Check sheet for the modelled part. Datum: model origin and axes. Units: mm. A direction names the side the tool comes from. Round coordinates to 2 decimals unless told otherwise and drop trailing zeros. Order: outer loops, then holes, each group sorted by start corner. A loop starts at its lowest first (then second) coordinate and runs counter-clockwise, first axis right, second up.
(1) Sectioned sample at C-C, the plane y = 14.75. Enter the section's corners in (x, z).
(2) Sectioned sample at B-B, the plane z = 0. Enter the section's corners in (x, y), and give its area (3 significant figures).
(3) Mould release check, pull along X, two halves, no side actions. Record for faces 3 (the cylindrical face through (15.51, -3.24, -3.44)), 4 (the flat face through (0, 0, 0)), 5 (the flat face through (7, -5.016, -13)): released by +X, released by -X, zero draft, split by the parting line, or undercut.
(4) Depth check by flat-ended pin: pin 1 (4 mm diameter, centred on x = 1.5, z = -4, fed in from +Y); pin 2 (6 mm diameter, centred on y = -0.5, z = 6, fed in from +X); pin 3 (6 mm diameter, centred on x = -7, z = -8, fed in from +Y); pin 4 (3 mm diameter, centred on x = -4, y = 9, fed in from -Z). Enter the tip coordinate at first touch or a pass-through.
(5) Tool access check on faces 1 (the flat face through (0, 15.899, 0)), 2 (the flat face through (11, -1.516, -11)). Record the directions out of +Z, -Z, +X, -X, +Y, -Y that give a thin tool (end or side, any length) a straight path to the whole face; none if there is none.
(6) Sectioned sample at D-D, the plane y = -2.5. Enter the section's corners in (x, z), and give its area (3 significant figures).
(7) Sectioned sample at A-A, the plane x = 0. Enter the section's corners in (y, z), and give its area (3 significant figures).
(8) Thickness scan on probe 1 along Y at (x, z) = (14, -5.5); probe 2 along Y at (x, z) = (-4, 1); probe 3 along X at (y, z) = (-0.25, -7.5). Record the ranges inside material, lowest first.
```python
from build123d import *

# Parameters (mm, degrees)
FILLET1_R     = 3
CHAMFER1_SIZE = 1
FILLET2_R     = 1


with BuildPart() as part:
    # Sketch1 → Revolve1 (revolve)
    with BuildSketch(Plane.XY, mode=Mode.PRIVATE) as revolve1_sk:
        Polygon((6, 10.999045222), (2.5, 10.999045222), (2.5, 15.899045222), (0, 15.899045222), (0, 3.5), (0, 0), (5.062177826, 0), (13.75, -5.015916471), (15.887822174, -5.015916471), (15.887822174, -1.515916471), (14.687822174, -1.515916471), (6, 3.5), align=None)
    revolve(revolve1_sk.sketch.rotate(Axis((0, 31.975823544, 0), (0, -1, 0)), 90), axis=Axis((0, 31.975823544, 0), (0, -1, 0)))

    # Fillet1
    fillet1_edges = [part.edges().sort_by_distance(p)[0] for p in [
        (0, -5.015916471, -13.75),
    ]]
    fillet(fillet1_edges, radius=FILLET1_R)

    # Chamfer1
    chamfer1_edges = [part.edges().sort_by_distance(p)[0] for p in [
        (0, 10.999045222, -6),
    ]]
    chamfer(chamfer1_edges, length=CHAMFER1_SIZE)

    # Fillet2
    fillet2_edges = [part.edges().sort_by_distance(p)[0] for p in [
        (0, -1.515916471, -14.687822174),
    ]]
    fillet(fillet2_edges, radius=FILLET2_R)


solid = part.part
```
Derived:
1. outline: circle Ø5 at (0, 0)
2. outline: (-15.89, -5.02) - (-14.55, -5.02) arc R3 ccw to (-13.05, -4.61) - (-5.06, 0) - (5.06, 0) - (13.05, -4.61) arc R3 ccw to (14.55, -5.02) - (15.89, -5.02) - (15.89, -1.52) - (14.96, -1.52) arc R1 cw to (14.46, -1.38) - (6, 3.5) - (6, 10) - (5, 11) - (2.5, 11) - (2.5, 15.9) - (-2.5, 15.9) - (-2.5, 11) - (-5, 11) - (-6, 10) - (-6, 3.5) - (-14.46, -1.38) arc R1 cw to (-14.96, -1.52) - (-15.89, -1.52) - close
2. area: 234 mm2
3. face 3: split by the parting line
3. face 4: undercut
3. face 5: zero draft
4. pin 1: stops at y = 15.9
4. pin 2: stops at x = 15.57
4. pin 3: stops at y = 2.56
4. pin 4: stops at z = -5.45
5. face 1: +Z, -Z, +X, -X, +Y
5. face 2: +Y
6. outline: circle Ø31.78 at (0, 0); hole circle Ø18.78 at (0, 0)
6. area: 516 mm2
7. outline: (-5.02, -15.89) - (-1.52, -15.89) - (-1.52, -14.96) arc R1 cw to (-1.38, -14.46) - (3.5, -6) - (10, -6) - (11, -5) - (11, -2.5) - (15.9, -2.5) - (15.9, 2.5) - (11, 2.5) - (11, 5) - (10, 6) - (3.5, 6) - (-1.38, 14.46) arc R1 cw to (-1.52, 14.96) - (-1.52, 15.89) - (-5.02, 15.89) - (-5.02, 14.55) arc R3 ccw to (-4.61, 13.05) - (0, 5.06) - (0, -5.06) - (-4.61, -13.05) arc R3 ccw to (-5.02, -14.55) - close
7. area: 234 mm2
8. probe 1: y = -5.02 to -1.52
8. probe 2: y = 0 to 11
8. probe 3: x = -9.99 to 9.99
